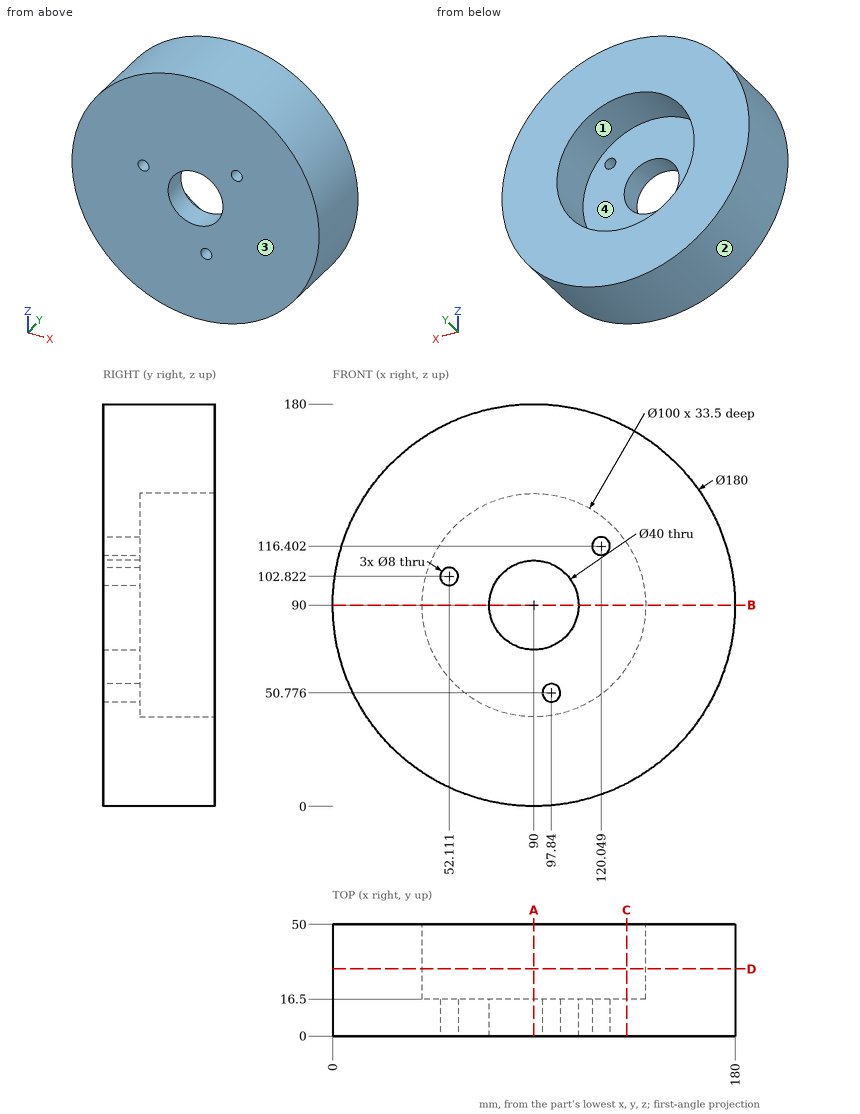
The figure shows three views and two pictorial views of one solid part (mm, origin at its lowest corner). Answer the questions. Coordinates: 2 decimals unless noted, no trailing zeros. Order: outer loops, then holes, each group sorted by start corner. A loop starts at its lowest first (then second) coordinate and runs counter-clockwise, first axis right, second up.
Q1. Given P1, Ø5, axis at x = 148.5, y = 23, coming from the +Z side (1 decimal); P2, Ø4, axis at y = 20.5, z = 119.5, coming from the -X side; P3, Ø5, axis at x = 136, y = 44.5, coming from the +Z side, each flat-ended and moving along its own axis, determine where each tip first touches the part or whether it passes through.
Q2. A cutting plane is placed at C-C, the plane x = 131.5. Write down the section's boundary in (y, z), and give its area (3 significant figures).
Q3. For a pull along Z with two mould halves and no side action, classify the marked faces 1, 2, 3 and 4 as pulls with the +Z half, pulls with the -Z half, needs draft (parallel to the pull), parting line crosses it, or undercut.
Q4. Consider line 1 (X direction, y = 36.5, z = 90); line 2 (Y direction, x = 131, z = 111); line 3 (X direction, y = 7, z = 75). Determine where each line is inside the solid, lowest interval first.
Q5. A cutting plane is placed at A-A, the plane x = 90. Write down the section's boundary in (y, z), and give its area (3 significant figures).
Q6. A cutting plane is placed at B-B, the plane z = 90. Write down the section's boundary in (x, y).
Q7. A cutting plane is placed at D-D, the plane y = 30. Write down the section's boundary in (x, z).
Answers follow:
1. P1: stops at z = 160.5
1. P2: stops at x = 4.3
1. P3: stops at z = 168.79
2. outline: (0, 10.14) - (50, 10.14) - (50, 62.11) - (16.5, 62.11) - (16.5, 117.89) - (50, 117.89) - (50, 169.86) - (0, 169.86) - close
2. area: 6,120 mm2
3. face 1: undercut
3. face 2: parting line crosses it
3. face 3: needs draft
3. face 4: undercut
4. line 1: x = 0 to 40, 140 to 180
4. line 2: y = 0 to 16.5
4. line 3: x = 1.26 to 76.77, 103.23 to 178.74
5. outline: (0, 0) - (50, 0) - (50, 40) - (16.5, 40) - (16.5, 70) - (0, 70) - close; (0, 110) - (16.5, 110) - (16.5, 140) - (50, 140) - (50, 180) - (0, 180) - close
5. area: 4,990 mm2
6. outline: (0, 0) - (70, 0) - (70, 16.5) - (40, 16.5) - (40, 50) - (0, 50) - close; (110, 0) - (180, 0) - (180, 50) - (140, 50) - (140, 16.5) - (110, 16.5) - close
7. outline: circle Ø180 at (90, 90); hole circle Ø100 at (90, 90)
